CAD build for the part. Positions are in the model's coordinates, mm. Face numbers are marked on the shaded views. A direction names the side the tool comes from. Round coordinates to 2 decimals unless told otherwise and drop trailing zeros. Loops run counter-clockwise (first coordinate to the right, second up) from the corner with the lowest first, then second, coordinate; pieces in that order, holes last. Notation, with made-up numbers: M -1,67 L 41,67 A31 ccw 41,100 Z; hole C 27.25,21.5 d6. An arc over 180 degrees is marked long. Use one line per item in the form item = value.
Autodesk Inventor part; units mm, degrees
ref_plane "YZ Plane" through (0, 0, 0) normal (1, 0, 0) x (0, 1, 0)
ref_plane "XZ Plane" through (0, 0, 0) normal (0, 1, 0) x (-1, 0, 0)
ref_plane "XY Plane" through (0, 0, 0) normal (0, 0, 1) x (1, 0, 0)
sketch "Sketch1" plane through (0, 0, 0) normal (0, 0, 1) x (1, 0, 0)
  circle A0 centre (0, 0) radius 10.795
  dimension "d0" = 21.59
extrude "Extrusion1" add sketch "Sketch1" along normal blind 6.35
fillet "Fillet1" radius 7.62 1 edges at (-10.795, 0, 6.35)
sketch "Sketch2" plane through (0, 0, 0) normal (0, 0, -1) x (-1, 0, 0)
  circle A0 centre (0, 0) radius 10.795
  circle A1 centre (0, 0) radius 5.715
  dimension "d4" = 11.43
extrude "Extrusion2" add sketch "Sketch2" against normal blind 11.43 contours A1
fillet "Fillet2" radius 1.905 1 edges at (5.715, 0, 11.43)
sketch "Sketch3" plane through (0, 0, 11.43) normal (0, 0, 1) x (1, 0, 0)
  line L0 (-0.6917, 1.5054) -> (0.568, 1.5054) construction
  line L1 (0.568, 1.5054) -> (0.568, -1.6512) construction
  line L2 (0.568, -1.6512) -> (-0.6917, -1.6512) construction
  line L3 (-0.6917, -1.6512) -> (-0.6917, 1.5054) construction
  spline S0 degree 2 poles (0.0592, -1.6512) (-0.0915, -1.6512) (-0.3409, -1.4512) (-0.4323, -1.2511) knots 0 0 0 1 2 2 2
  spline S1 degree 2 poles (-0.4323, -1.2511) (-0.5237, -1.0535) (-0.625, -0.4607) (-0.625, -0.0754) knots 0 0 0 1 2 2 2
  spline S2 degree 2 poles (-0.625, -0.0754) (-0.625, 0.3075) (-0.5287, 0.8756) (-0.4348, 1.0855) knots 0 0 0 1 2 2 2
  spline S3 degree 2 poles (-0.4348, 1.0855) (-0.3434, 1.2905) (-0.0939, 1.5054) (0.0617, 1.5054) knots 0 0 0 1 2 2 2
  spline S4 degree 2 poles (0.0617, 1.5054) (0.1382, 1.5054) (0.2741, 1.461) (0.3309, 1.4264) knots 0 0 0 1 2 2 2
  spline S5 degree 2 poles (0.3309, 1.4264) (0.3803, 1.3943) (0.484, 1.3029) (0.5334, 1.2485) knots 0 0 0 1 2 2 2
  line L4 (0.5334, 1.2485) -> (0.5334, 0.7595)
  line L5 (0.5334, 0.7595) -> (0.5162, 0.7595)
  spline S6 degree 2 poles (0.5162, 0.7595) (0.4915, 0.8089) (0.405, 0.9472) (0.3457, 1.0139) knots 0 0 0 1 2 2 2
  spline S7 degree 2 poles (0.3457, 1.0139) (0.2864, 1.0781) (0.1506, 1.1596) (0.0592, 1.1596) knots 0 0 0 1 2 2 2
  spline S8 degree 2 poles (0.0592, 1.1596) (-0.0371, 1.1596) (-0.2125, 0.9991) (-0.2792, 0.8459) knots 0 0 0 1 2 2 2
  spline S9 degree 2 poles (-0.2792, 0.8459) (-0.3434, 0.6903) (-0.415, 0.2186) (-0.415, -0.0754) knots 0 0 0 1 2 2 2
  spline S10 degree 2 poles (-0.415, -0.0754) (-0.415, -0.3891) (-0.3385, -0.8411) (-0.2743, -0.9967) knots 0 0 0 1 2 2 2
  spline S11 degree 2 poles (-0.2743, -0.9967) (-0.21, -1.1474) (-0.0371, -1.3005) (0.0592, -1.3005) knots 0 0 0 1 2 2 2
  spline S12 degree 2 poles (0.0592, -1.3005) (0.1481, -1.3005) (0.2963, -1.2141) (0.3556, -1.1498) knots 0 0 0 1 2 2 2
  spline S13 degree 2 poles (0.3556, -1.1498) (0.4124, -1.0856) (0.4939, -0.9522) (0.5186, -0.9053) knots 0 0 0 1 2 2 2
  line L6 (0.5186, -0.9053) -> (0.5334, -0.9053)
  line L7 (0.5334, -0.9053) -> (0.5334, -1.3894)
  spline S14 degree 2 poles (0.5334, -1.3894) (0.484, -1.4364) (0.3951, -1.5228) (0.3309, -1.5623) knots 0 0 0 1 2 2 2
  spline S15 degree 2 poles (0.3309, -1.5623) (0.2642, -1.6068) (0.1506, -1.6512) (0.0592, -1.6512) knots 0 0 0 1 2 2 2
extrude "Extrusion3" cut sketch "Sketch3" against normal blind 0.0635
sketch "Sketch4" plane through (0, 0, 0) normal (0, 0, -1) x (-1, 0, 0)
  circle A0 centre (0, 0) radius 10.795
extrude "Extrusion4" cut sketch "Sketch4" against normal blind 0.635
properties part number "C Stick"
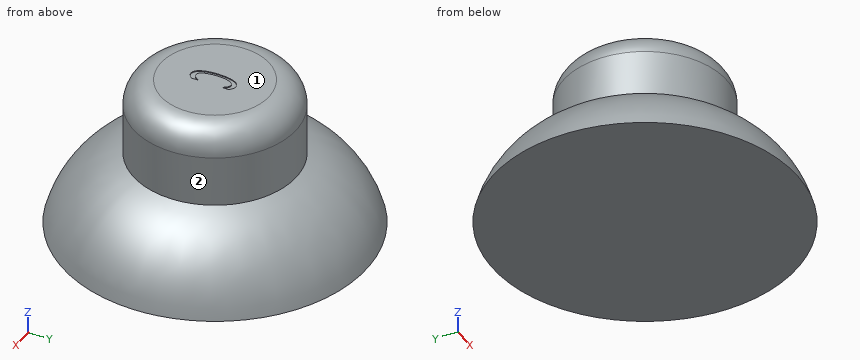
1. Drop flat-ended pins along their axis: P1, Ø5, axis at y = -7, z = 7, coming from the +X side; P2, Ø2, axis at x = 3, y = -8, coming from the +Z side; P3, Ø5, axis at x = -1.5, z = 4.5, coming from the -Y side. Give the stop position or say it passes through.
Completed:
P1 = 5.33
P2 = 5.05
P3 = -10.09
2. Probe line 1 along X through (y, z) = (3.5, 3.75); line 2 along Z through (x, y) = (3.25, 4.25) (3 decimals); line 3 along Z through (x, y) = (8.75, -0.5) (3 decimals). List the from-to ranges inside material, lowest first. Write a range as from..to.
Completed:
line_1 = -8.31..8.31
line_2 = 0.635..10.646
line_3 = 0.635..4.022
3. Tool access for the marked faces 1 and 2: list every direction of +Z, -Z, +X, -X, +Y, -Y with a clear straight run to the whole face (end or side of a thin tool).
Completed:
face_1 = +Z, +X, -X, +Y, -Y
face_2 = +Z
4. Cut at A-A on z = 8.25. Write the cut outline in (x, y) (3 decimals).
Completed:
outline = C 0,0 d11.43
